Build history of the part. All positions in model axes, mm. A direction names the side the tool comes from. Coordinates: 2 decimals unless noted, no trailing zeros. Loops run counter-clockwise (first coordinate to the right, second up) from the corner with the lowest first, then second, coordinate; pieces in that order, holes last.
(1) Slice it at C-C (x = -22). Give the cut face in (y, z).
(2) Slice it at D-D (x = 2.5). Give the cut face in (y, z).
(3) Slice it at A-A (y = 7.25). Give the cut face in (x, z).
(4) Wall check: L1, parallel to Y at x = -39, z = 8; L2, parallel to Z at x = -18, y = 14; L3, parallel to Y at x = -22.5, z = -11.5. Give the ranges that are in metal, low to high.
(5) Flat gauge pins, fed straight in: P1, Ø5, axis at x = -27, y = 9.5, coming from the +Z side; P2, Ø1, axis at y = 2, z = -2.5, coming from the -X side; P3, Ø8, axis at x = -37, y = 11.5, coming from the -Z side. Where does each tip first touch, or does it go through?
(6) Slice it at B-B (z = 1.5). Give the cut face in (x, y).
(7) Tool access for faces 1 (the face through (-40, 2, 0)), 2 (the face through (-30, 11, 10)), 3 (the face through (-31, 11, -10)), 4 (the face through (-35, 11, 0)): list every direction of +Z, -Z, +X, -X, +Y, -Y with a clear straight run to the whole face (end or side of a thin tool).
(8) Two-plate mould, pull along Y, no slides. Class faces 5 (the face through (-1, 2, -14)), 6 (the face through (-40, 18.2, 0)), 7 (the face through (-43, 3.2, 0)): pulls with the +Y half, pulls with the -Y half, needs draft (parallel to the pull), parting line crosses it, or undercut.
Autodesk Inventor part; units mm, degrees
ref_plane "YZ Plane" through (0, 0, 0) normal (1, 0, 0) x (0, 1, 0)
ref_plane "XZ Plane" through (0, 0, 0) normal (0, 1, 0) x (-1, 0, 0)
ref_plane "XY Plane" through (0, 0, 0) normal (0, 0, 1) x (1, 0, 0)
sketch "Boceto1" plane through (0, 0, 0) normal (0, 1, 0) x (-1, 0, 0)
  line L0 (-40, 14) -> (40, 14)
  line L1 (40, 14) -> (40, -14)
  line L2 (40, -14) -> (-40, -14)
  line L3 (-40, -14) -> (-40, 14)
  line L4 (-40, 14) -> (40, -14) construction
  line L5 (40, 14) -> (-40, -14) construction
  point P0 (0, 0)
  dimension "d0" = 80
  dimension "d1" = 28
extrude "Extrusión1" add sketch "Boceto1" along normal blind 3.2
sketch "Boceto2" plane through (0, 3.2, 0) normal (0, 1, 0) x (1, 0, 0)
  line L0 (-45, 10) -> (-16, 10)
  line L1 (-16, 10) -> (-16, -10)
  line L2 (-16, -10) -> (-45, -10)
  line L3 (-45, -10) -> (-45, 10)
  line L4 (-45, 10) -> (-16, -10) construction
  line L5 (-16, 10) -> (-45, -10) construction
  line L6 (-40, 14) -> (-40, -14)
  point P0 (0, 0)
  point P1 (-30.5, 0)
  dimension "d4" = 20
  dimension "d5" = 29
  dimension "d6" = 5
extrude "Extrusión2" add sketch "Boceto2" along normal blind 16
sketch "Boceto3" plane through (-45, 3.2, -10) normal (-1, 0, 0) x (0, 0, 1)
  line L0 (-4, 0) -> (0, 0)
  line L1 (20, 0) -> (20, 16)
  line L2 (1, 1) -> (19, 1)
  line L3 (19, 1) -> (19, 15)
  line L4 (19, 15) -> (1, 15)
  line L5 (1, 15) -> (1, 1)
  line L6 (1, 1) -> (19, 15) construction
  line L7 (19, 1) -> (1, 15) construction
  point P0 (10, -3.2)
  point P1 (0, 16)
  point P2 (10, 8)
  dimension "d9" = 18
  dimension "d10" = 14
extrude "Extrusión3" cut sketch "Boceto3" against normal blind 10
properties part number "ESP32_PoE"
Response values:
1. outline: (0, -14) - (3.2, -14) - (3.2, -10) - (19.2, -10) - (19.2, 10) - (3.2, 10) - (3.2, 14) - (0, 14) - close
2. outline: (0, -14) - (3.2, -14) - (3.2, 14) - (0, 14) - close
3. outline: (-45, -10) - (-16, -10) - (-16, 10) - (-45, 10) - (-45, 9) - (-35, 9) - (-35, -9) - (-45, -9) - close
4. L1: y = 0 to 4.2, 18.2 to 19.2
4. L2: z = -10 to 10
4. L3: y = 0 to 3.2
5. P1: stops at z = 10
5. P2: stops at x = -40
5. P3: stops at z = -10
6. outline: (-45, 3.2) - (-40, 3.2) - (-40, 0) - (40, 0) - (40, 3.2) - (-16, 3.2) - (-16, 19.2) - (-45, 19.2) - (-45, 18.2) - (-35, 18.2) - (-35, 4.2) - (-45, 4.2) - close
7. face 1: +Z, -Z, -X, -Y
7. face 2: +Z, +X, -X, +Y
7. face 3: -Z, +X, -X, +Y
7. face 4: -X
8. face 5: needs draft
8. face 6: undercut
8. face 7: pulls with the -Y half
